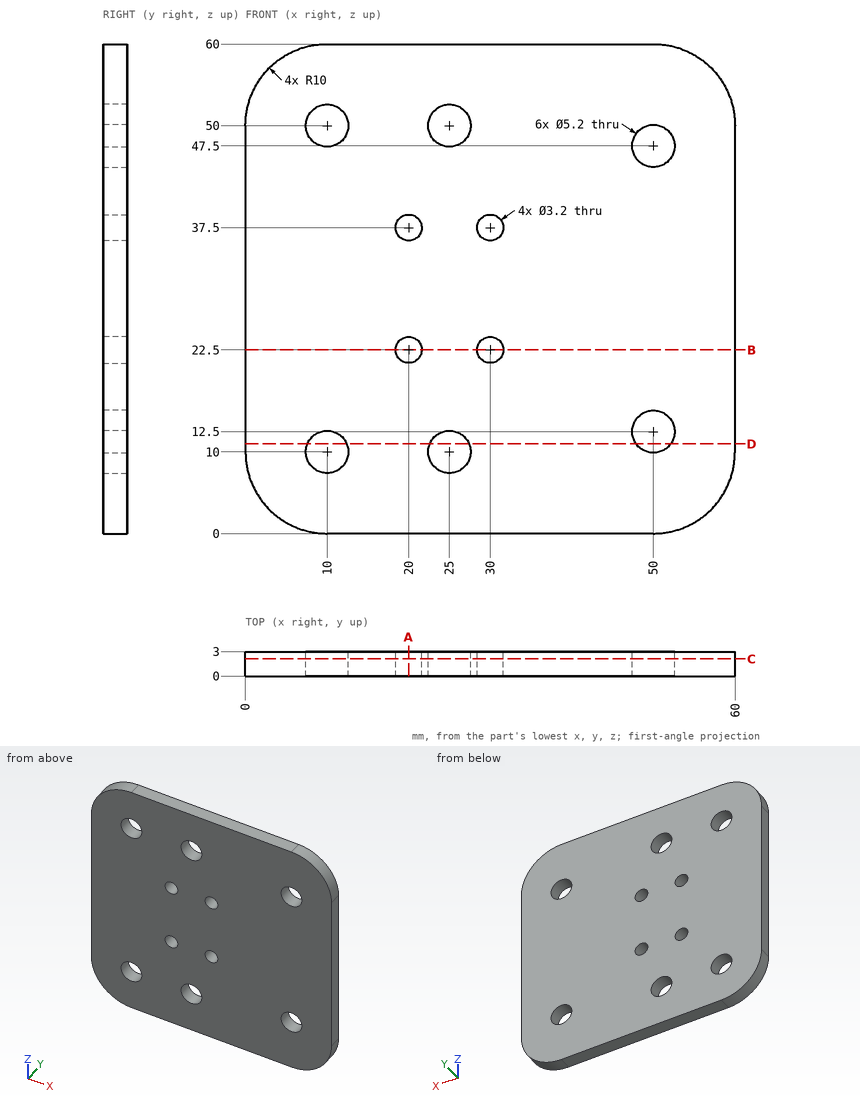
Answer from the drawing. Dimensions are ordinates in mm from the lowest x, y and z of the part. Coordinates: 2 decimals unless noted, no trailing zeros. Write each loop counter-clockwise with the first axis right and the second up, starting at its lowest first coordinate (ties: lowest second). Pieces come first, ordered by that corner, then holes. Notation, with made-up numbers: (84.25, 75.5) - (93.25, 75.5) arc R17 cw to (93.25, 81.5) - close; hole circle Ø11 at (50, 33). An arc over 180 degrees is marked (long way). Return JSON: item names as keys, results as strings. Group by question number.
Q1. The part is cut by section D-D on z = 11. Write down the section's boundary in (x, y).
Q2. The part is cut by section C-C on y = 2.1. State how many separate pieces and enclosed holes the cut face has, and give its area (3 significant figures).
Q3. Find the intervals of material crossed by line 1 along X through (y, z) = (1.25, 37.5); line 2 along Z through (x, y) = (31, 0.25); line 3 along X through (y, z) = (0.55, 8), in increasing order. Write a range as [from, to].
Q4. A flat-ended cylindrical pin translates along its axis: pin 1 Ø3 at (x, z) = (30, 37.5) entering from -Y. Find the tip coordinate at first contact, or state that the pin passes through.
Q5. The part is cut by section B-B on z = 22.5. Write down the section's boundary in (x, y), and give its area (3 significant figures).
Q6. The part is cut by section A-A on x = 20. Write down the section's boundary in (y, z), and give its area (3 significant figures).
Evaluation:
{
 "1": {"outline": "(0, 0) - (7.6, 0) - (7.6, 3) - (0, 3) - close; (12.4, 0) - (22.6, 0) - (22.6, 3) - (12.4, 3) - close; (27.4, 0) - (47.88, 0) - (47.88, 3) - (27.4, 3) - close; (52.12, 0) - (60, 0) - (60, 3) - (52.12, 3) - close"},
 "2": {"separate pieces": "1", "enclosed holes": "10", "area": "3,350 mm2"},
 "3": {"line 1": "x = [0, 18.4], [21.6, 28.4], [31.6, 60]", "line 2": "z = [0, 21.25], [23.75, 36.25], [38.75, 60]", "line 3": "x = [0.2, 8.34], [11.66, 23.34], [26.66, 59.8]"},
 "4": {"pin 1": "passes through"},
 "5": {"outline": "(0, 0) - (18.4, 0) - (18.4, 3) - (0, 3) - close; (21.6, 0) - (28.4, 0) - (28.4, 3) - (21.6, 3) - close; (31.6, 0) - (60, 0) - (60, 3) - (31.6, 3) - close", "area": "161 mm2"},
 "6": {"outline": "(0, 0) - (3, 0) - (3, 20.9) - (0, 20.9) - close; (0, 24.1) - (3, 24.1) - (3, 35.9) - (0, 35.9) - close; (0, 39.1) - (3, 39.1) - (3, 60) - (0, 60) - close", "area": "161 mm2"}
}
